Read the model definition and answer for the solid it produces. Units are mm, in the model's axes. A direction names the side the tool comes from. Round coordinates to 2 decimals unless told otherwise and drop trailing zeros. Write each loop counter-clockwise with the first axis right and the second up, starting at its lowest first coordinate (ties: lowest second). Pieces come first, ordered by that corner, then holes. Notation, with made-up numbers: (-22, 31.25) -> (31, 31.25) arc R31 ccw to (31, 61.25) -> close; hole circle Ø4 at (76.25, -26.5). An arc over 180 degrees is marked (long way). Return JSON: item names as keys, results as strings. Group by question number.
(1) A cutting plane is placed at D-D on x = 1.5. Give the vertices of the cut face in (y, z).
(2) For faces 4 (the cylindrical face through (1.05, 3.77, -31.34)), 5 (the flat face through (0, 3, 0)), 6 (the flat face through (-7.5, 2, 1)), determine the directions among +Z, -Z, +X, -X, +Y, -Y from which every point of the face is accessible in a straight line to the end or side of a thin tool.
(3) The mould has two halves that part along X. Classify faces 1 (the flat face through (-2, 2.5, 30)), 2 (the flat face through (-2, 0, -1)), 3 (the flat face through (7.5, 2, -29)): released by +X, released by -X, zero draft, split by the parting line, or undercut.
(4) A cutting plane is placed at B-B on z = -28. Give the vertices of the cut face in (x, y), then the cut area to 3 significant figures.
(5) A cutting plane is placed at A-A on x = 5.5. Give the vertices of the cut face in (y, z), then the cut area to 3 significant figures.
(6) Straight lines are drawn through the part: line 1 (X direction, y = 1.3, z = 28); line 2 (Z direction, x = -3, y = 2.75); line 3 (X direction, y = 3.45, z = -28). For each, find the intervals that lie inside material, in ascending order.
(7) A cutting plane is placed at C-C on y = 3.25. Give the vertices of the cut face in (x, z), then the cut area to 3 significant figures.
(8) Given pin 1 (2 mm diameter, centred on x = 1.5, z = 27.5, fed in from +Y), flat-ended and moving along its own axis, determine where the tip first touches the part or whether it passes through.
```python
from build123d import *

# Parameters (mm, degrees)
SKETCH1_W           = 15
SKETCH1_H           = 80
BOSS_EXTRUDE1_DEPTH = 5
SKETCH2_R           = 3.5
CUT_EXTRUDE1_DEPTH  = 2.5
FILLET1_R           = 1
SKETCH3_W           = 7.5
SKETCH3_H           = 35
CUT_EXTRUDE2_DEPTH  = 42.003048667
SKETCH4_R           = 2.5
CUT_EXTRUDE3_DEPTH  = 41.773766076


with BuildPart() as part:
    # Sketch1 → Boss-Extrude1 (new body)
    with BuildSketch(Plane(origin=(0, 0, 0), x_dir=(1, 0, 0), z_dir=(0, 1, 0))):
        Rectangle(SKETCH1_W, SKETCH1_H)
    extrude(amount=BOSS_EXTRUDE1_DEPTH)

    # Sketch2 → Cut-Extrude1 (cut)
    with BuildSketch(Plane(origin=(0, 5, 0), x_dir=(1, 0, 0), z_dir=(0, 1, 0))):
        with Locations(Location((0, -28, 0), (0, 0, 270))):
            Circle(SKETCH2_R)
    cut_extrude1 = extrude(amount=-CUT_EXTRUDE1_DEPTH, mode=Mode.SUBTRACT)

    # Mirror1: Cut-Extrude1 across plane
    add(cut_extrude1.mirror(Plane.XY), mode=Mode.SUBTRACT)

    # Fillet1
    fillet1_edges = [part.edges().sort_by_distance(p)[0] for p in [
        (-7.5, 5, 0),
        (0, 5, 40),
        (7.5, 5, 0),
        (0, 5, -40),
    ]]
    fillet(fillet1_edges, radius=FILLET1_R)

    # Sketch3 → Cut-Extrude2 (cut, through all)
    with BuildSketch(Plane(origin=(0, 5, 0), x_dir=(1, 0, 0), z_dir=(0, 1, 0))):
        with Locations((3.75, 0)):
            Rectangle(SKETCH3_W, SKETCH3_H)
    extrude(amount=-CUT_EXTRUDE2_DEPTH, mode=Mode.SUBTRACT)

    # Sketch4 → Cut-Extrude3 (cut, through all)
    with BuildSketch(Plane(origin=(0, 2.5, 0), x_dir=(1, 0, 0), z_dir=(0, 1, 0))):
        with Locations(Location((0, 28, 0), (0, 0, 270))):
            Circle(SKETCH4_R)
        with Locations(Location((0, -28, 0), (0, 0, 270))):
            Circle(SKETCH4_R)
    extrude(amount=-CUT_EXTRUDE3_DEPTH, mode=Mode.SUBTRACT)


solid = part.part
```
Checks:
{
 "1": {"outline": "(0, -40) -> (4, -40) arc R1 ccw to (5, -39) -> (5, -31.16) -> (2.5, -31.16) -> (2.5, -30) -> (0, -30) -> close; (0, -26) -> (2.5, -26) -> (2.5, -24.84) -> (5, -24.84) -> (5, -17.5) -> (0, -17.5) -> close; (0, 17.5) -> (5, 17.5) -> (5, 24.84) -> (2.5, 24.84) -> (2.5, 26) -> (0, 26) -> close; (0, 30) -> (2.5, 30) -> (2.5, 31.16) -> (5, 31.16) -> (5, 39) arc R1 ccw to (4, 40) -> (0, 40) -> close"},
 "2": {"face 4": "+Y", "face 5": "+X, +Y, -Y", "face 6": "+Z, -Z, -X, +Y, -Y"},
 "3": {"face 1": "undercut", "face 2": "zero draft", "face 3": "released by +X"},
 "4": {"outline": "(-7.5, 0) -> (-2.5, 0) -> (-2.5, 2.5) -> (-3.5, 2.5) -> (-3.5, 5) -> (-6.5, 5) arc R1 ccw to (-7.5, 4) -> close; (2.5, 0) -> (7.5, 0) -> (7.5, 4) arc R1 ccw to (6.5, 5) -> (3.5, 5) -> (3.5, 2.5) -> (2.5, 2.5) -> close", "area": "44.6 mm^2"},
 "5": {"outline": "(0, -40) -> (4, -40) arc R1 ccw to (5, -39) -> (5, -17.5) -> (0, -17.5) -> close; (0, 17.5) -> (5, 17.5) -> (5, 39) arc R1 ccw to (4, 40) -> (0, 40) -> close", "area": "225 mm^2"},
 "6": {"line 1": "x = -7.5 to -2.5, 2.5 to 7.5", "line 2": "z = -40 to -29.8, -26.2 to 26.2, 29.8 to 40", "line 3": "x = -7.5 to -3.5, 3.5 to 7.5"},
 "7": {"outline": "(-7.5, -40) -> (7.5, -40) -> (7.5, -17.5) -> (0, -17.5) -> (0, 17.5) -> (7.5, 17.5) -> (7.5, 40) -> (-7.5, 40) -> close; hole circle Ø7 at (0, -28); hole circle Ø7 at (0, 28)", "area": "861 mm^2"},
 "8": {"pin 1": "stops at y = 2.5"}
}
